Could you check a few things on this drawing? It's one solid part, dimensions in mm from its lowest x, y, z. Round coordinates to 2 decimals unless told otherwise and drop trailing zeros. Write each loop counter-clockwise with the first axis right and the second up, starting at its lowest first coordinate (ties: lowest second). Pieces come first, ordered by that corner, then holes. Notation, with made-up numbers: M -13,-22.5 L 34,-22.5 A28 cw 34,7.5 Z; hole C -10,-27.5 d8. An arc over 180 degrees is marked long. One line per item, written item: value. Start each with the question number.
(1) I want a section at B-B on x = 3. Please give me the cut outline in (y, z), and give its area (3 significant figures).
(2) I'm going to push flat-ended pins straight in: pin 1 Ø2.5 at (x, z) = (3, 27) entering from +Y; pin 2 Ø4 at (x, z) = (91, 27) entering from +Y; pin 3 Ø0.9 at (y, z) = (5, 19) entering from -X; pin 4 Ø2 at (x, y) = (84, 4.5) entering from +Z. Where does each tip first touch, or does it pass through?
(3) I want a section at D-D on x = 68. Please give me the cut outline in (y, z), and give its area (3 significant figures).
(4) If I drill on L1, parallel to X at y = 1.65, z = 27; L2, parallel to Y at x = 48, z = 4; L3, parallel to Z at x = 10, y = 4.55, over which ranges is the centre line in solid material (lowest first)?
(5) I want a section at C-C on z = 20. Please give me the cut outline in (x, y).
(6) I want a section at A-A on z = 3. Please give me the cut outline in (x, y), and give its area (3 significant figures).
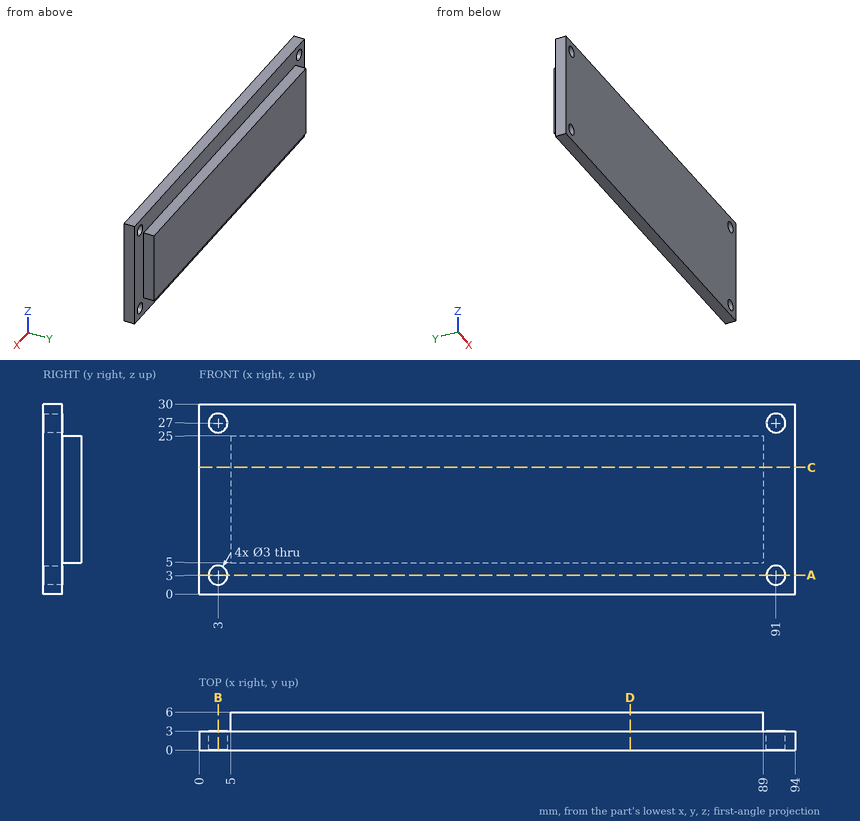
Found:
1. outline: M 0,0 L 3,0 L 3,1.5 L 0,1.5 Z; M 0,4.5 L 3,4.5 L 3,25.5 L 0,25.5 Z; M 0,28.5 L 3,28.5 L 3,30 L 0,30 Z
1. area: 72.0 mm²
2. pin 1: passes through
2. pin 2: stops at y = 3
2. pin 3: stops at x = 5
2. pin 4: stops at z = 25
3. outline: M 0,0 L 3,0 L 3,5 L 6,5 L 6,25 L 3,25 L 3,30 L 0,30 Z
3. area: 150 mm²
4. L1: x = 0 to 1.5, 4.5 to 89.5, 92.5 to 94
4. L2: y = 0 to 3
4. L3: z = 5 to 25
5. outline: M 0,0 L 94,0 L 94,3 L 89,3 L 89,6 L 5,6 L 5,3 L 0,3 Z
6. outline: M 0,0 L 1.5,0 L 1.5,3 L 0,3 Z; M 4.5,0 L 89.5,0 L 89.5,3 L 4.5,3 Z; M 92.5,0 L 94,0 L 94,3 L 92.5,3 Z
6. area: 264 mm²
